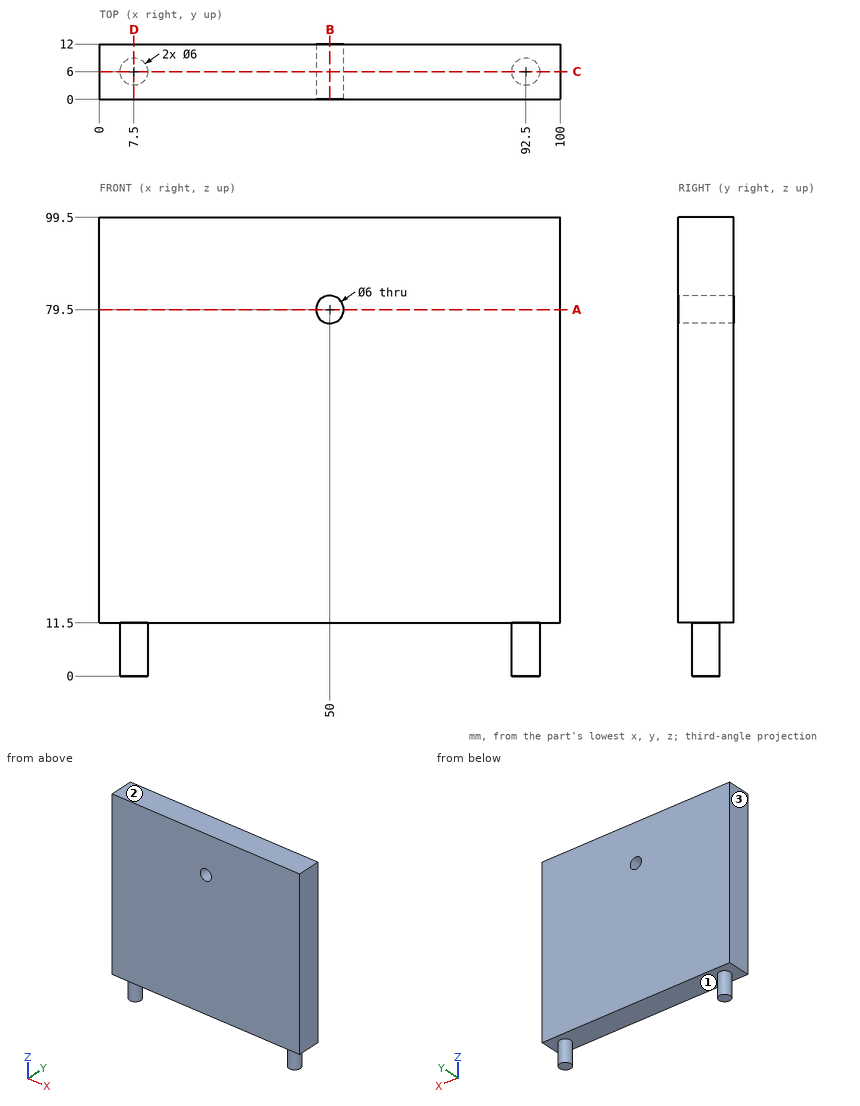
Verification items for this drawing (mm, ordinates from the low corner). Coordinates: 2 decimals unless noted, no trailing zeros. Loops run counter-clockwise (first coordinate to the right, second up) from the corner with the lowest first, then second, coordinate; pieces in that order, holes last.
Item 1: Thickness scan on line 1 (Z direction, x = 50, y = 7); line 2 (Z direction, x = 36, y = 2.75); line 3 (X direction, y = 8.25, z = 8.5). Record the ranges inside material, lowest first.
Item 2: Go/stop test with a flat-tipped pin: pin 1 Ø6 at (x, y) = (78.5, 5) entering from -Z. Record where the tip stops, or that it passes through.
Item 3: Release check for a two-part mould opening along X. For the marked faces 1, 2 and 3 record: released by +X, released by -X, zero draft, split by the parting line, or undercut.
Item 4: Sectioned sample at B-B, the plane x = 50. Record the boundary of the cut face in (y, z), then the cut area to 3 significant figures.
Item 5: Sectioned sample at C-C, the plane y = 6. Record the boundary of the cut face in (x, z), then the cut area to 3 significant figures.
Item 6: Sectioned sample at D-D, the plane x = 7.5. Record the boundary of the cut face in (y, z).
Item 7: Sectioned sample at A-A, the plane z = 79.5. Record the boundary of the cut face in (x, y).
Check result:
1. line 1: z = 11.5 to 76.5, 82.5 to 99.5
1. line 2: z = 11.5 to 99.5
1. line 3: x = 5.52 to 9.48, 90.52 to 94.48
2. pin 1: stops at z = 11.5
3. face 1: undercut
3. face 2: zero draft
3. face 3: released by -X
4. outline: (0, 11.5) - (12, 11.5) - (12, 76.5) - (0, 76.5) - close; (0, 82.5) - (12, 82.5) - (12, 99.5) - (0, 99.5) - close
4. area: 984 mm2
5. outline: (0, 11.5) - (4.5, 11.5) - (4.5, 0) - (10.5, 0) - (10.5, 11.5) - (89.5, 11.5) - (89.5, 0) - (95.5, 0) - (95.5, 11.5) - (100, 11.5) - (100, 99.5) - (0, 99.5) - close; hole circle Ø6 at (50, 79.5)
5. area: 8,910 mm2
6. outline: (0, 11.5) - (3, 11.5) - (3, 0) - (9, 0) - (9, 11.5) - (12, 11.5) - (12, 99.5) - (0, 99.5) - close
7. outline: (0, 0) - (47, 0) - (47, 12) - (0, 12) - close; (53, 0) - (100, 0) - (100, 12) - (53, 12) - close
